Autodesk Inventor part; units mm, degrees
ref_plane "YZ Plane" through (0, 0, 0) normal (1, 0, 0) x (0, 1, 0)
ref_plane "XZ Plane" through (0, 0, 0) normal (0, 1, 0) x (-1, 0, 0)
ref_plane "XY Plane" through (0, 0, 0) normal (0, 0, 1) x (1, 0, 0)
sketch "Sketch1" plane through (0, 0, 0) normal (0, 1, 0) x (-1, 0, 0)
  circle A0 centre (0, 0) radius 11
  line L0 (0, 0) -> (0, -24.9996)
  line L1 (12.5, 17) -> (-12.5, 17)
  line L2 (-12.5, 17) -> (-12.5, -41)
  line L3 (-12.5, -41) -> (12.5, -41)
  line L4 (12.5, -41) -> (12.5, 17)
  circle A1 centre (0, 0) radius 8.5
  line L5 (0, 11) -> (9.8279, 11) construction
  line L6 (0, -11) -> (10.2574, -11) construction
  dimension "d0" = 22
  dimension "d1" = 2.5
  dimension "d2" = 25
  dimension "d3" = 6
  dimension "d4" = 30
extrude "Extrusion1" add sketch "Sketch1" along normal mid plane 12 contours A0 | L4 L3 L2 L1
extrude "Extrusion2" cut sketch "Sketch1" along normal mid plane 7.2 contours A0
sketch "Sketch2" plane through (-12.5, 6, 17) normal (0, 0, 1) x (1, 0, 0)
  line L0 (1.5, -9.6) -> (1.5, -2.4)
  line L1 (23.5, -9.6) -> (23.5, -2.4)
  line L2 (23.5, -2.4) -> (1.5, -2.4)
  line L3 (1.5, -9.6) -> (23.5, -9.6)
  point P0 (12.5, -6)
ref_plane "Work Plane1" through (0, 0, 0) normal (0, 0, 1) x (1, 0, 0)
extrude "Extrusion3" cut sketch "Sketch2" against normal up to surface (17 mm away)
ref_plane "Work Plane2" through (0, 0, 11) normal (0, 0, 1) x (1, 0, 0)
sketch "Sketch3" plane through (12.5, -6, -41) normal (1, 0, 0) x (0, 0, -1)
  line L0 (-52, -2.4) -> (-52, 14.4) construction
  circle A0 centre (-53.6, 6) radius 1.6
  point P0 (-41, 6)
  dimension "d11" = 3.2
extrude "Extrusion4" cut sketch "Sketch3" against normal through all
sketch "Sketch4" plane through (12.5, 6, -41) normal (0, 0, -1) x (-1, 0, 0)
  line L0 (22, -3) -> (3, -3)
  line L1 (3, -3) -> (3, -9)
  line L2 (3, -9) -> (22, -9)
  line L3 (22, -9) -> (22, -3)
  line L4 (0, 0) -> (25, 0)
  line L5 (25, -12) -> (0, -12)
  line L6 (25, -12) -> (25, 0)
  line L7 (0, -12) -> (0, 0)
  point P0 (12.5, -6)
  dimension "d14" = 3
  dimension "d15" = 3
  dimension "d16" = 3
  dimension "d17" = 3
extrude "Extrusion5" cut sketch "Sketch4" against normal blind 25 contours L3 L2 L1 L0
sketch "Sketch7" plane through (0, 6, 0) normal (0, 1, 0) x (1, 0, 0)
  line L0 (-9.5, 41) -> (-9.5, 16)
  line L1 (9.5, 41) -> (9.5, 16)
  line L2 (-9.5, 16) -> (9.5, 16)
  line L3 (9.5, 16) -> (9.5, 36)
  line L4 (9.5, 36) -> (-9.5, 36)
  line L5 (-9.5, 36) -> (-9.5, 16)
  line L6 (12.5, 41) -> (-12.5, 41)
  point P0 (0, 0)
  dimension "d20" = 5
extrude "Extrusion6" cut sketch "Sketch7" against normal through all contours L4 L1 L2 L0
sketch "Sketch8" plane through (12.5, -6, -41) normal (1, 0, 0) x (0, 0, -1)
  circle A0 centre (-10, 6) radius 1.5
  circle A1 centre (-20, 6) radius 1.5
  line L0 (0, 0) -> (0, 12)
  point P0 (-41, 6)
  dimension "d23" = 3
  dimension "d24" = 3
  dimension "d25" = 10
  dimension "d26" = 10
extrude "Extrusion7" cut sketch "Sketch8" against normal through all
properties part number "connecting_rod_crankschaft_side"
Can you work these out from the model? Positions are in its coordinate system, mm. A direction names the side the tool comes from. Coordinates: 2 decimals unless noted, no trailing zeros. Loops run counter-clockwise (first coordinate to the right, second up) from the corner with the lowest first, then second, coordinate; pieces in that order, holes last. Notation, with made-up numbers: M 7,63.25 L 42,63.25 A22 ccw 42,99.25 Z; hole C 82.5,31 d11. An arc over 180 degrees is marked long. Return JSON: item names as keys, results as strings. Group by question number.
Item 1: Imagine slicing it at D-D (y = -5). Please give me the cut outline in (x, z), and give its area (3 significant figures).
Item 2: Imagine slicing it at C-C (z = 12.6). Please give me the cut outline in (x, y), and give its area (3 significant figures).
Item 3: On a 3-axis mill with a long thin cutter (end or side, diameter ignored), from which of +Z, -Z, +X, -X, +Y, -Y can I reach the whole of each face in a straight line? I mean faces 5 (the flat face through (9.5, 0, -29)), 6 (the flat face through (0, 5, -36)), 7 (the flat face through (-11, 0, 9)), 8 (the flat face through (0, 3, -39)). Say none if no direction works.
Item 4: Imagine slicing it at A-A (x = 0). Please give me the cut outline in (y, z), and give its area (3 significant figures).
Item 5: If I drill on L1, parallel to Z at x = 0, y = 4.6; L2, parallel to X at y = 4.5, z = -29; L3, parallel to Y at x = -12.15, z = 12.6, over which ranges is the centre line in solid material (lowest first)? Write a range as from..to.
Item 6: Imagine slicing it at B-B (z = -31). Please give me the cut outline in (x, y), and give its area (3 significant figures).
Item 7: Thinking about a two-plate mould opening in Y: for faces 1 (the flat face through (0, 6, -12)), 2 (the cylindrical face through (11.02, 0.07, -29.5)), 3 (the flat face through (0, -4, -36)), 4 (the flat face through (0, -3.6, 9)), which applies, released by +Y, released by -Y, zero draft, split by the parting line, or undercut?
Item 8: I'm going to push a flat-ended pin straight in: pin 1 Ø13.5 at (x, z) = (0, 0) entering from +Y (3 decimals). Where does the tip first touch, or does it pass through?
Verdict:
{
 "1": {"outline": "M -12.5,-41 L 12.5,-41 L 12.5,17 L -12.5,17 Z; hole M -9.5,-36 L 9.5,-36 L 9.5,-16 L -9.5,-16 Z; hole C 0,0 d17", "area": "843 mm^2"},
 "2": {"outline": "M -12.5,-6 L 12.5,-6 L 12.5,-1.6 L 11,-1.6 L 11,-3.6 L -11,-3.6 L -11,-1.6 L -12.5,-1.6 Z; M -12.5,1.6 L -11,1.6 L -11,3.6 L 11,3.6 L 11,1.6 L 12.5,1.6 L 12.5,6 L -12.5,6 Z", "area": "132 mm^2"},
 "3": {"face 5": "none", "face 6": "+Y, -Y", "face 7": "+Z", "face 8": "-Z"},
 "4": {"outline": "M -6,-41 L -3,-41 L -3,-36 L -6,-36 Z; M -6,-16 L 6,-16 L 6,-8.5 L 3.6,-8.5 L 3.6,-11 L -3.6,-11 L -3.6,-8.5 L -6,-8.5 Z; M -6,8.5 L -3.6,8.5 L -3.6,17 L -6,17 Z; M 3,-41 L 6,-41 L 6,-36 L 3,-36 Z; M 3.6,8.5 L 6,8.5 L 6,17 L 3.6,17 Z", "area": "143 mm^2"},
 "5": {"L1": "z = -41..-36, -16..-8.5, 8.5..17", "L2": "x = -12.5..-9.5, 9.5..12.5", "L3": "y = -6..-1.6, 1.6..6"},
 "6": {"outline": "M -12.5,-6 L -9.5,-6 L -9.5,-1.5 L -12.5,-1.5 Z; M -12.5,1.5 L -9.5,1.5 L -9.5,6 L -12.5,6 Z; M 9.5,-6 L 12.5,-6 L 12.5,-1.5 L 9.5,-1.5 Z; M 9.5,1.5 L 12.5,1.5 L 12.5,6 L 9.5,6 Z", "area": "54.0 mm^2"},
 "7": {"face 1": "released by +Y", "face 2": "undercut", "face 3": "zero draft", "face 4": "undercut"},
 "8": {"pin 1": "passes through"}
}
